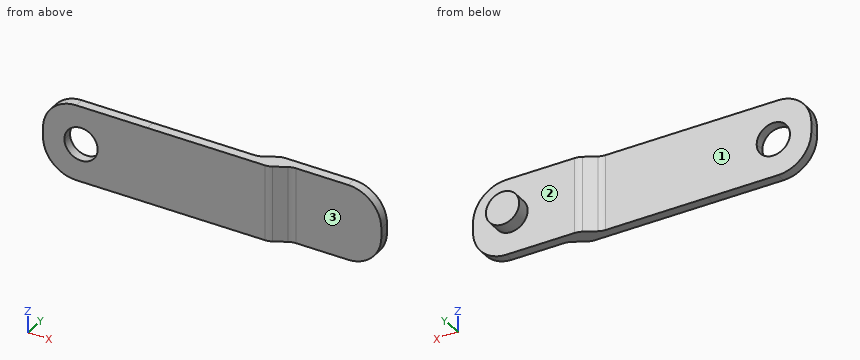
from build123d import *

# Parameters (mm, degrees)
BOSS_EXTRUDE1_DEPTH = 4
SKETCH4_W           = 7
SKETCH4_H           = 2
CUT_EXTRUDE2_DEPTH  = 17.000717669
FILLET1_R           = 3
SKETCH5_R           = 3.5
BOSS_EXTRUDE2_DEPTH = 3


with BuildPart() as part:
    # Sketch1 → Boss-Extrude1 (new body)
    with BuildSketch(Plane(origin=(0, 0, 0), x_dir=(1, 0, 0), z_dir=(0, 1, 0))):
        with BuildLine():
            Line((35.408940815, -1.068857927), (35.408963598, 0.931142073))
            ThreePointArc((35.408963598, 0.931142073), (33.358767452, 5.880912897), (28.40904334, 7.931221814))
            Line((28.40904334, 7.931221814), (-12.665132622, 7.931689714))
            Line((-12.665132622, 7.931689714), (-27.590956657, 7.931859742))
            ThreePointArc((-27.590956657, 7.931859742), (-32.54072748, 5.881663596), (-34.591036397, 0.931939484))
            Line((-34.591036397, 0.931939484), (-34.591059181, -1.068060516))
            ThreePointArc((-34.591059181, -1.068060516), (-32.540863035, -6.01783134), (-27.591138922, -8.068140257))
            Line((-27.591138922, -8.068140257), (-12.665314887, -8.068310285))
            Line((-12.665314887, -8.068310285), (28.408861074, -8.068778185))
            ThreePointArc((28.408861074, -8.068778185), (33.358631898, -6.018582039), (35.408940815, -1.068857927))
        make_face()
        with BuildLine():
            ThreePointArc((27.408912336, -3.568766794), (30.908952207, -0.068806665), (27.408992077, 3.431233206))
            ThreePointArc((27.408992077, 3.431233206), (23.908952207, -0.068726924), (27.408912336, -3.568766794))
        make_face(mode=Mode.SUBTRACT)
        with BuildLine():
            ThreePointArc((-23.09104779, -0.068191519), (-26.591007919, 3.431848351), (-30.091047789, -0.068111778))
            ThreePointArc((-30.091047789, -0.068111778), (-26.59108766, -3.568151649), (-23.09104779, -0.068191519))
        make_face(mode=Mode.SUBTRACT)
        with BuildLine():
            ThreePointArc((27.408992077, 3.431233206), (23.908952207, -0.068726924), (27.408912336, -3.568766794))
            ThreePointArc((27.408912336, -3.568766794), (30.908952207, -0.068806665), (27.408992077, 3.431233206))
        make_face()
    extrude(amount=BOSS_EXTRUDE1_DEPTH)

    # Sketch4 → Cut-Extrude2 (cut, through all)
    with BuildSketch(Plane(origin=(-9.1912e-05, 0, 8.068454562), x_dir=(1, 0, 1.1392e-05), z_dir=(-1.1392e-05, 0, 1))):
        Polygon((9.464868883, 2), (13.271442145, 4), (-27.591047011, 4), (-27.591047011, 2), align=None)
        with Locations((-31.091047011, 3)):
            Rectangle(SKETCH4_W, SKETCH4_H)
        Polygon((28.408952989, 0), (28.408952989, 2), (16.665047436, 2), (12.858474174, 0), align=None)
        with Locations((31.908952989, 1)):
            Rectangle(SKETCH4_W, SKETCH4_H)
    extrude(amount=-CUT_EXTRUDE2_DEPTH, mode=Mode.SUBTRACT)

    # Fillet1
    fillet1_edges = [part.edges().sort_by_distance(p)[0] for p in [
        (12.858473393, 0, 0.068601041),
        (13.271441364, 4, 0.068605746),
        (16.665046655, 2, 0.068644404),
        (9.464868102, 2, 0.068562383),
    ]]
    fillet(fillet1_edges, radius=FILLET1_R)

    # Sketch5 → Boss-Extrude2 (add)
    with BuildSketch(Plane(origin=(0, 4, 0), x_dir=(1, 0, 0), z_dir=(0, 1, 0))):
        with Locations((27.408952207, -0.068766794)):
            Circle(SKETCH5_R)
    extrude(amount=BOSS_EXTRUDE2_DEPTH)


solid = part.part
Design review of the part built by this model. Coordinates are the model's own, in mm. Face numbers are marked on the shaded views. A direction names the side the tool comes from. Give positions to 0.01 mm unless a question says otherwise; leave off trailing zeros. Write each loop counter-clockwise with the first axis right and the second up, starting at its lowest first coordinate (ties: lowest second). Pieces come first, ordered by that corner, then holes. Notation, with made-up numbers: M 80,40.5 L 133,40.5 A26 ccw 133,71.5 Z; hole C 47,59.5 d2. An arc over 180 degrees is marked long. Answer as a JSON object with one key per item and string values. Group by question number.
1) Tool access review of the marked faces 1, 2 and 3: name each direction out of +Z, -Z, +X, -X, +Y, -Y from which nothing blocks a thin tool from reaching the whole face with its end or side.
2) We need section B-B (y = 3). Give the boundary of the cut face in (x, z).
3) We need section C-C (x = -9). Give the boundary of the cut face in (y, z), and give its area (3 significant figures).
4) Clearance check with flat-ended pins moving along their axes: pin 1 Ø8 at (x, z) = (13, 2.5) entering from +Y; pin 2 Ø5 at (x, z) = (24, -3.5) entering from -Y; pin 3 Ø8 at (x, z) = (-19, -2.5) entering from +Y. State where each tip first meets the part, or that it passes through.
5) For line 1 along Y through (x, z) = (1, -4.5); line 2 along Y through (x, z) = (23, -4); line 3 along X through (y, z) = (1.75, -2.5), list the stretches that pass through material, from the lowest coordinate up.
6) We need section A-A (x = -27). Give the boundary of the cut face in (y, z), and give its area (3 significant figures).
Answer key:
{
 "1": {"face 1": "+Z, -Z, -X, +Y", "face 2": "+Y", "face 3": "+Z, -Z, +X, -Y"},
 "2": {"outline": "M 11.37,-7.93 L 28.41,-7.93 A7 ccw 35.41,-0.93 L 35.41,1.07 A7 ccw 28.41,8.07 L 11.37,8.07 Z"},
 "3": {"outline": "M 0,-7.93 L 2,-7.93 L 2,8.07 L 0,8.07 Z", "area": "32.0 mm²"},
 "4": {"pin 1": "stops at y = 4", "pin 2": "stops at y = 2", "pin 3": "stops at y = 2"},
 "5": {"line 1": "y = 0 to 2", "line 2": "y = 2 to 4", "line 3": "x = -34.41 to -28.97, -24.21 to 16.21"},
 "6": {"outline": "M 0,-7.93 L 2,-7.93 L 2,-3.41 L 0,-3.41 Z; M 0,3.54 L 2,3.54 L 2,8.07 L 0,8.07 Z", "area": "18.1 mm²"}
}
